The model under review builds one solid part; all positions refer to its coordinate system, in mm. Give positions to 0.01 mm unless a question says otherwise; leave off trailing zeros. Write each loop counter-clockwise with the first axis right and the second up, starting at its lowest first coordinate (ties: lowest second). Pieces come first, ordered by that corner, then holes. Notation, with made-up numbers: (-6.5, 2) - (30.5, 2) arc R27 cw to (30.5, 29) - close; hole circle Ø5 at (-2.5, -32). An arc over 180 degrees is marked (long way). Write item = value, one per line.
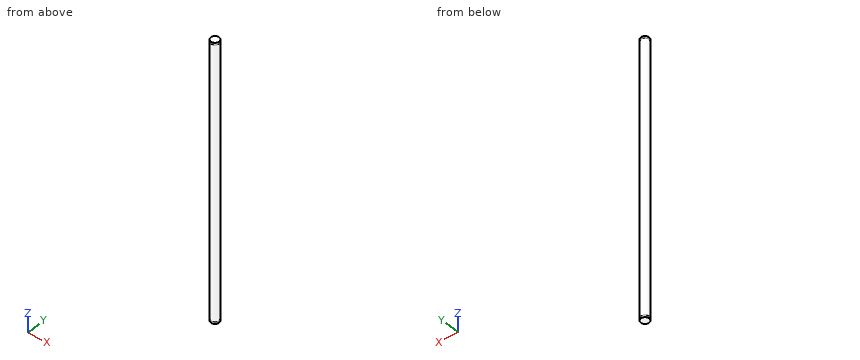
```python
from build123d import *

# Parameters (mm, degrees)
TORUS001_R     = 2
TORUS_R        = 2
CYLINDER_R     = 5.75
CYLINDER_DEPTH = 383


with BuildPart() as torus001:
    # Torus001 → Torus001 (revolve)
    with BuildSketch(Plane(origin=(0, 0, 381), x_dir=(1, 0, 0), z_dir=(0, -1, 0))):
        with Locations((7.5, 0)):
            Circle(TORUS001_R)
    revolve(axis=Axis((0, 0, 381), (0, 0, 1)))


with BuildPart() as torus:
    # Torus → Torus (revolve)
    with BuildSketch(Plane(origin=(0, 0, 2), x_dir=(1, 0, 0), z_dir=(0, -1, 0))):
        with Locations((7.5, 0)):
            Circle(TORUS_R)
    revolve(axis=Axis((0, 0, 2), (0, 0, 1)))


with BuildPart() as cut001:
    # Cylinder → Cylinder (new body)
    with BuildSketch(Plane.XY):
        Circle(CYLINDER_R)
    extrude(amount=CYLINDER_DEPTH)

    # Cut: cut Torus
    add(torus.part, mode=Mode.SUBTRACT)

    # Cut001: cut Torus001
    add(torus001.part, mode=Mode.SUBTRACT)


solid = cut001.part
```
1. Insertion check: P1, Ø3, axis at x = -4, z = 157.5, coming from the -Y side; P2, Ø3, axis at x = 1, z = 264, coming from the -Y side; P3, Ø3, axis at y = 2.5, z = 128, coming from the -X side; P4, Ø2, axis at y = -3.5, z = 215, coming from the -X side. Each pin has a flat end and moves straight along its axis. Give the tip position at first contact, or say it passes through.
Findings below:
P1 = -5.18
P2 = -5.75
P3 = -5.66
P4 = -5.18
2. For line 1 (Y direction, x = -0.75, z = 140); line 2 (Y direction, x = -3.25, z = 246); line 3 (X direction, y = -3.5, z = 130.5), list the stretches that pass through material, from the lowest coordinate up. Write a range as from..to.
Findings below:
line_1 = -5.7..5.7
line_2 = -4.74..4.74
line_3 = -4.56..4.56
3. Take a section at A-A on z = 184. Give the boundary of the cut face in (x, y).
Findings below:
outline = circle Ø11.5 at (0, 0)
